from build123d import *

# Parameters (mm, degrees)
SKETCH_1_R      = 0.5
EXTRUDE_1_DEPTH = 1
EXTRUDE_START   = -2.45
EXTRUDE_2_DEPTH = 2.45
FILLET_1_R      = 0.2


with BuildPart() as part:
    # 草图1 → 凸台-拉伸1 (new body)
    with BuildSketch(Plane.XY):
        with BuildLine():
            Line((-14.016792693, -2.096749739), (-6.313489141, -2.525837459))
            ThreePointArc((-6.313489141, -2.525837459), (-6.8, 0), (-6.313489141, 2.525837459))
            Line((-6.313489141, 2.525837459), (-14.016792693, 2.096749739))
            ThreePointArc((-14.016792693, 2.096749739), (-16, 0), (-14.016792693, -2.096749739))
        make_face()
        with Locations((-10.3, 0)):
            Circle(SKETCH_1_R, mode=Mode.SUBTRACT)
        with Locations((-14.3, 0)):
            Circle(SKETCH_1_R, mode=Mode.SUBTRACT)
        with Locations((-8.3, 0)):
            Circle(SKETCH_1_R, mode=Mode.SUBTRACT)
        with Locations((-12.3, 0)):
            Circle(SKETCH_1_R, mode=Mode.SUBTRACT)
    extrude(amount=EXTRUDE_1_DEPTH)

    # 草图3 → 凸台-拉伸2 (add)
    with BuildSketch(Plane.XY.offset(1).offset(EXTRUDE_START)):
        with BuildLine():
            Line((-6.313489141, 4.028162673), (-14.100216045, 3.594428124))
            ThreePointArc((-14.100216045, 3.594428124), (-17.5, 0), (-14.100216045, -3.594428124))
            Line((-14.100216045, -3.594428124), (-6.313489141, -4.028162673))
            Line((-6.313489141, -4.028162673), (-6.313489141, -2.525837459))
            Line((-6.313489141, -2.525837459), (-14.016792693, -2.096749739))
            ThreePointArc((-14.016792693, -2.096749739), (-16, 0), (-14.016792693, 2.096749739))
            Line((-14.016792693, 2.096749739), (-6.313489141, 2.525837459))
            Line((-6.313489141, 2.525837459), (-6.313489141, 4.028162673))
        make_face()
    extrude(amount=EXTRUDE_2_DEPTH)

    # 圆角1
    fillet_1_edges = [part.edges().sort_by_distance(p)[0] for p in [
        (-10.206852593, 3.811295398, 1),
        (-17.5, 0, 1),
        (-10.206852593, -3.811295398, 1),
        (-17.5, 0, -1.45),
        (-10.206852593, -3.811295398, -1.45),
        (-6.313489141, -4.028162673, -0.225),
        (-6.313489141, 4.028162673, -0.225),
        (-10.206852593, 3.811295398, -1.45),
    ]]
    fillet(fillet_1_edges, radius=FILLET_1_R)


solid = part.part
Here's how the part is built. I have some questions about the finished solid (model axes, mm). A direction names the side the tool comes from. Coordinates: 2 decimals unless noted, no trailing zeros. Loops run counter-clockwise (first coordinate to the right, second up) from the corner with the lowest first, then second, coordinate; pieces in that order, holes last. Notation, with made-up numbers: (74, 44) -> (108, 44) arc R18 ccw to (108, 78) -> close; hole circle Ø9 at (49.25, 55.25). An arc over 180 degrees is marked (long way). Use one line per item in the form item = value. Start each with the question number.
(1) Will these pins go through, and if not, where does the flat tip stop? pin 1 (2 mm diameter, centred on x = -9, y = -1, fed in from -Z); pin 2 (1 mm diameter, centred on x = -15, z = 0.5, fed in from -Y).
(2) If we section it at A-A (z = 0.6): Please give me the cut outline in (x, y).
(3) We'd pull the mould along X, two halves only. Please class faces 1 (the face through (-6.313, -3, 0)), 2 (the face through (-10.4, -3.8, -0.2)), 3 (the face through (-8.8, 0, 0.5)), 4 (the face through (-11.9, -2.5, -1.45)): pulls with the +X half, pulls with the -X half, needs draft (parallel to the pull), parting line crosses it, or undercut.
(4) On a 3-axis mill with a long thin cutter (end or side, diameter ignored), from which of +Z, -Z, +X, -X, +Y, -Y can I reach the whole of each face in a straight line? I mean faces 5 (the face through (-16, 0, -1)), 6 (the face through (-11.838, -0.192, 0.493)). Say none if no direction works.
(5) Please list where these lines run through material, in increasing order: line 1 along Z through (x, y) = (-13.5, 1); line 2 along Y through (x, z) = (-12.3, 0.6); line 3 along Y through (x, z) = (-8.3, 0.75).
Verdict:
q1.pin_1 = 0
q1.pin_2 = -3.55
q2.outline = (-14.1, -3.59) -> (-6.52, -4.02) arc R0.2 ccw to (-6.31, -3.82) -> (-6.31, -2.53) arc R6.8 cw to (-6.31, 2.53) -> (-6.31, 3.82) arc R0.2 ccw to (-6.52, 4.02) -> (-14.1, 3.59) arc R3.6 ccw to start; hole circle Ø1 at (-14.3, 0); hole circle Ø1 at (-12.3, 0); hole circle Ø1 at (-10.3, 0); hole circle Ø1 at (-8.3, 0)
q3.face_1 = pulls with the +X half
q3.face_2 = pulls with the -X half
q3.face_3 = undercut
q3.face_4 = needs draft
q4.face_5 = -Z, +X
q4.face_6 = +Z, -Z
q5.line_1 = 0 to 1
q5.line_2 = -3.69 to -0.5, 0.5 to 3.69
q5.line_3 = -3.92 to -0.5, 0.5 to 3.92
